Design review of the part built by this model. Coordinates are the model's own, in mm. A direction names the side the tool comes from. Give positions to 0.01 mm unless a question says otherwise; leave off trailing zeros. Write each loop counter-clockwise with the first axis right and the second up, starting at its lowest first coordinate (ties: lowest second). Pieces come first, ordered by that corner, then holes. Notation, with made-up numbers: M -5,2 L 18,2 A21 cw 18,19 Z; hole C -19.75,-24.75 d8. An arc over 180 degrees is marked long. Answer in a Markdown table with one row per item.
Autodesk Inventor part; units mm, degrees
ref_plane "YZ Plane" through (0, 0, 0) normal (1, 0, 0) x (0, 1, 0)
ref_plane "XZ Plane" through (0, 0, 0) normal (0, 1, 0) x (-1, 0, 0)
ref_plane "XY Plane" through (0, 0, 0) normal (0, 0, 1) x (1, 0, 0)
sketch "Block1" plane through (0, 0, 0) normal (0, 0, 1) x (1, 0, 0)
  circle A0 centre (74.029, 24.2723) radius 1
  line L0 (49.279, 30.4723) -> (71.779, 30.4723)
  line L1 (71.779, 30.4723) -> (71.779, 18.0723)
  line L2 (71.779, 18.0723) -> (49.279, 18.0723)
  line L3 (49.279, 18.0723) -> (49.279, 30.4723)
  line L4 (49.279, 30.4723) -> (44.779, 30.4723)
  line L5 (44.779, 30.4723) -> (44.779, 18.0723)
  line L6 (44.779, 18.0723) -> (49.279, 18.0723)
  line L7 (49.279, 18.0723) -> (49.279, 30.4723)
  line L8 (71.779, 30.4723) -> (76.279, 30.4723)
  line L9 (76.279, 30.4723) -> (76.279, 18.0723)
  line L10 (76.279, 18.0723) -> (71.779, 18.0723)
  line L11 (71.779, 18.0723) -> (71.779, 30.4723)
  line L12 (44.779, 24.2723) -> (76.279, 24.2723) construction
  line L13 (47.029, 30.4723) -> (47.029, 18.0723) construction
  circle A1 centre (47.029, 24.2723) radius 1
  line L14 (74.029, 30.4723) -> (74.029, 18.0723) construction
  point P0 (60.979, 24.0984)
  dimension "d7" = 22.5
  dimension "d8" = 12.4
  dimension "d9" = 4.5
  dimension "d10" = 4.5
  dimension "d11" = 2
  dimension "d12" = 2
sketch "Sketch1" plane through (0, 0, 0) normal (0, 0, 1) x (1, 0, 0)
  line L0 (-38.4282, 40.714) -> (0.0718, 40.714)
  line L1 (0.0718, 40.714) -> (0.0718, 33.714)
  line L2 (0.0718, 33.714) -> (-38.4282, 33.714)
  line L3 (-38.4282, 33.714) -> (-38.4282, 40.714)
  line L4 (-92.7646, -8.503) -> (-89.7646, -8.503)
  line L5 (-89.7646, -8.503) -> (-89.7646, -11.753)
  line L6 (-89.7646, -11.753) -> (-92.7646, -11.753)
  line L7 (-92.7646, -11.753) -> (-92.7646, -8.503)
  line L8 (-92.7646, -21.6527) -> (-89.7646, -21.6527)
  line L9 (-89.7646, -21.6527) -> (-89.7646, -21.7527)
  line L10 (-89.7646, -21.7527) -> (-92.7646, -21.7527)
  line L11 (-92.7646, -21.7527) -> (-92.7646, -21.6527)
  line L12 (-32.6782, 33.714) -> (-5.6782, 33.714)
  line L13 (-5.6782, 33.714) -> (-5.6782, -16.286)
  line L14 (-5.6782, -16.286) -> (-32.6782, -16.286)
  line L15 (-32.6782, -16.286) -> (-32.6782, 33.714)
  line L16 (-19.1782, 40.714) -> (-19.1782, 33.714) construction
  line L17 (-19.1782, -16.286) -> (-19.1782, 33.714) construction
  line L18 (-35.9282, 23.714) -> (-32.6782, 23.714)
  line L19 (-32.6782, 23.714) -> (-32.6782, 9.714)
  line L20 (-32.6782, 9.714) -> (-35.9282, 9.714)
  line L21 (-35.9282, 9.714) -> (-35.9282, 23.714)
  line L22 (-2.4282, 23.714) -> (-5.6782, 23.714)
  line L23 (-5.6782, 23.714) -> (-5.6782, 9.714)
  line L24 (-5.6782, 9.714) -> (-2.4282, 9.714)
  line L25 (-2.4282, 9.714) -> (-2.4282, 23.714)
  line L26 (-35.9282, -2.286) -> (-32.6782, -2.286)
  line L27 (-32.6782, -2.286) -> (-32.6782, -16.286)
  line L28 (-32.6782, -16.286) -> (-35.9282, -16.286)
  line L29 (-35.9282, -16.286) -> (-35.9282, -2.286)
  line L30 (-2.4282, -2.286) -> (-5.6782, -2.286)
  line L31 (-5.6782, -2.286) -> (-5.6782, -16.286)
  line L32 (-5.6782, -16.286) -> (-2.4282, -16.286)
  line L33 (-2.4282, -16.286) -> (-2.4282, -2.286)
  line L34 (-21.6782, -16.286) -> (-16.6782, -16.286)
  line L35 (-16.6782, -16.286) -> (-16.6782, -19.536)
  line L36 (-16.6782, -19.536) -> (-21.6782, -19.536)
  line L37 (-21.6782, -19.536) -> (-21.6782, -16.286)
  line L38 (-19.1782, -16.286) -> (-19.1782, -19.536) construction
  point P0 (0, 0)
  dimension "d0" = 3
  dimension "mat" = 3.25
  dimension "d2" = 3
  dimension "d3" = 0.1
  dimension "d4" = 38.5
  dimension "d6" = 7
  dimension "d17" = 27
  dimension "d20" = 50
  dimension "d23" = 3.25
  dimension "d24" = 14
  dimension "d25" = 10
  dimension "d26" = 3.25
  dimension "d27" = 14
  dimension "d28" = 5
  dimension "d29" = 3.25
extrude "Extrusion2" add sketch "Sketch1" along normal blind 3.25 contours L0 L1 L2 L3 | L2 L13 L14 L15 | L15 L20 L21 L18 | L22 L25 L24 L13 | L15 L28 L29 L26 | L30 L33 L32 L13 | L14 L35 L36 L37
equation "\"d23\" = mat"
equation "\"d26\" = mat"
equation "\"d29\" = mat"
equation "\"d30\" = mat"
properties part number "arm-servo"
1) Add section D-D (y = 30). Write out the cut boundary in (x, z).
Geometry says:
| item | result |
|---|---|
| outline | M -32.68,0 L -5.68,0 L -5.68,3.25 L -32.68,3.25 Z |
2) Add section C-C (y = -5). Write out the cut boundary in (x, z), and give its area (3 significant figures).
Geometry says:
| item | result |
|---|---|
| outline | M -35.93,0 L -2.43,0 L -2.43,3.25 L -35.93,3.25 Z |
| area | 109 mm^2 |
3) Add section B-B (z = 2.25). Write out the cut boundary in (x, y).
Geometry says:
| item | result |
|---|---|
| outline | M -38.43,33.71 L -32.68,33.71 L -32.68,23.71 L -35.93,23.71 L -35.93,9.71 L -32.68,9.71 L -32.68,-2.29 L -35.93,-2.29 L -35.93,-16.29 L -21.68,-16.29 L -21.68,-19.54 L -16.68,-19.54 L -16.68,-16.29 L -2.43,-16.29 L -2.43,-2.29 L -5.68,-2.29 L -5.68,9.71 L -2.43,9.71 L -2.43,23.71 L -5.68,23.71 L -5.68,33.71 L 0.07,33.71 L 0.07,40.71 L -38.43,40.71 Z |
4) The part is to be moulded in two halves that separate along Y. For faces 1 (the face through (0.072, 37, 2)), 2 (the face through (-19, 40.714, 2)), 3 (the face through (-5.678, 29, 2)), say which applies: released by +Y, released by -Y, zero draft, split by the parting line, or undercut.
Geometry says:
| item | result |
|---|---|
| face 1 | zero draft |
| face 2 | released by +Y |
| face 3 | undercut |
5) To check wall thickness, follow probe 1 along Y at (x, z) = (-2.5, 0.5); probe 2 along X at (y, z) = (31.5, 2.65); probe 3 along X at (y, z) = (15, 0.2). State the ranges of each line that lie inside material, in increasing order. Write a range as [from, to].
Geometry says:
| item | result |
|---|---|
| probe 1 | [-16.29, -2.29], [9.71, 23.71], [33.71, 40.71] |
| probe 2 | [-32.68, -5.68] |
| probe 3 | [-35.93, -2.43] |
6) For faces 4 (the face through (-16.678, -18, 2)), 5 (the face through (-4, 9.714, 2)), 6 (the face through (-34, 9.714, 2)), 7 (the face through (-29, -16.286, 2)), list the 3-axis set-ups (+Z, -Z, +X, -X, +Y, -Y) from which the entire face can be reached by the end or side of a thin tool; tool diameter is ignored.
Geometry says:
| item | result |
|---|---|
| face 4 | +Z, -Z, +X, -Y |
| face 5 | +Z, -Z, +X |
| face 6 | +Z, -Z, -X |
| face 7 | +Z, -Z, -X, -Y |
7) Add section A-A (x = -34). Write out the cut boundary in (y, z), and give its area (3 significant figures).
Geometry says:
| item | result |
|---|---|
| outline | M -16.29,0 L -2.29,0 L -2.29,3.25 L -16.29,3.25 Z; M 9.71,0 L 23.71,0 L 23.71,3.25 L 9.71,3.25 Z; M 33.71,0 L 40.71,0 L 40.71,3.25 L 33.71,3.25 Z |
| area | 114 mm^2 |
8) Insertion check: P1, Ø1, axis at x = -26.5, z = 2.5, coming from the -Y side; P2, Ø1.6, axis at y = -7, z = 1, coming from the +X side; P3, Ø1.6, axis at y = 3, z = 1.5, coming from the -X side. Each pin has a flat end and moves straight along its axis. Give the tip position at first contact, or say it passes through.
Geometry says:
| item | result |
|---|---|
| P1 | y = -16.29 |
| P2 | x = -2.43 |
| P3 | x = -32.68 |
